Could you check a few things on this model? Use its own coordinates, in mm. Round coordinates to 2 decimals unless told otherwise and drop trailing zeros. Loops run counter-clockwise (first coordinate to the right, second up) from the corner with the lowest first, then second, coordinate; pieces in that order, holes last. Notation, with made-up numbers: (12.5, 26.25) -> (55.5, 26.25) arc R16 ccw to (55.5, 50.25) -> close; hole circle Ø6 at (15.5, 49). An arc over 180 degrees is marked (long way). Write each question's results on one line, items separated by ' | '.
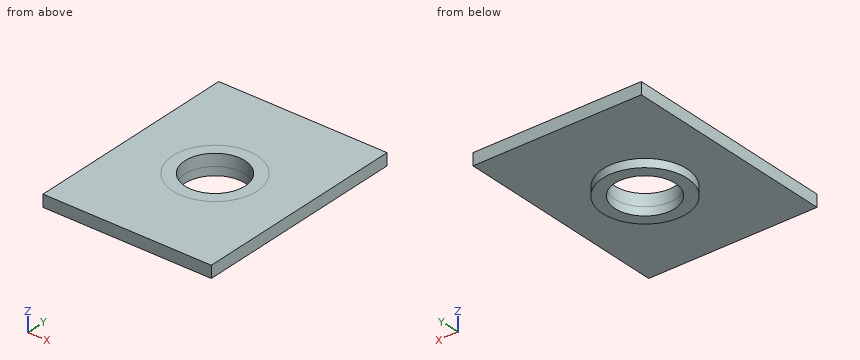
from build123d import *

# Parameters (mm, degrees)
CROQUIS1_R              = 35
SALIENTE_EXTRUIR1_DEPTH = 10
CROQUIS2_R              = 35
CROQUIS2_R_2            = 25
SALIENTE_EXTRUIR2_DEPTH = 7
SALIENTE_EXTRUIR4_START = -10
CROQUIS3_R              = 35
CROQUIS3_R_2            = 25
SALIENTE_EXTRUIR4_DEPTH = 10


with BuildPart() as part:
    # Croquis1 → Saliente-Extruir1 (new body)
    with BuildSketch(Plane.XY):
        Polygon((0, 0), (140, 0), (140, 180), (0, 180), (0, 49.177666069), align=None)
        with Locations((70, 90)):
            Circle(CROQUIS1_R, mode=Mode.SUBTRACT)
    extrude(amount=SALIENTE_EXTRUIR1_DEPTH)



with BuildPart() as body_2:
    # Croquis2 → Saliente-Extruir2 (new body)
    with BuildSketch(Plane(origin=(0, 0, 0), x_dir=(-1, 0, 0), z_dir=(0, 0, -1))):
        with Locations(Location((-70, 90, 0), (0, 0, 180))):
            Circle(CROQUIS2_R)
        with Locations((-70, 90)):
            Circle(CROQUIS2_R_2, mode=Mode.SUBTRACT)
    extrude(amount=SALIENTE_EXTRUIR2_DEPTH)


with BuildPart() as part_1:
    add(part.part)

    add(body_2.part)  # Saliente-Extruir4 merges body 2
    # Croquis3 → Saliente-Extruir4 (add)
    with BuildSketch(Plane.XY.offset(10).offset(SALIENTE_EXTRUIR4_START)):
        with Locations((70, 90)):
            Circle(CROQUIS3_R)
        with Locations((70, 90)):
            Circle(CROQUIS3_R_2, mode=Mode.SUBTRACT)
    extrude(amount=SALIENTE_EXTRUIR4_DEPTH)


solid = part_1.part
1) I want a section at C-C, the plane z = 2.75. Write out the boundary of the cut face in (x, y), plus the area to 3 significant figures.
Model answer:
outline: (0, 0) -> (140, 0) -> (140, 180) -> (0, 180) -> close; hole circle Ø50 at (70, 90) | area: 23,200 mm2
2) I'm going to push a flat-ended pin straight in: pin 1 (3 mm diameter, centred on x = 110.5, y = 91, fed in from -Z). Where does the tip first touch, or does it pass through?
Model answer:
pin 1: stops at z = 0
3) I want a section at D-D, the plane y = 62. Write out the boundary of the cut face in (x, z).
Model answer:
outline: (0, 0) -> (49, 0) -> (49, -7) -> (91, -7) -> (91, 0) -> (140, 0) -> (140, 10) -> (0, 10) -> close
4) I want a section at A-A, the plane y = 90. Write out the boundary of the cut face in (x, z).
Model answer:
outline: (0, 0) -> (35, 0) -> (35, -7) -> (45, -7) -> (45, 10) -> (0, 10) -> close; (95, -7) -> (105, -7) -> (105, 0) -> (140, 0) -> (140, 10) -> (95, 10) -> close
5) I need wall thicknesses on line 1 (X direction, y = 90, z = 7.75); line 2 (Y direction, x = 70, z = -2.25); line 3 (Z direction, x = 13.5, y = 149). Which ranges of each line are inside material? Lowest first, please.
Model answer:
line 1: x = 0 to 45, 95 to 140 | line 2: y = 55 to 65, 115 to 125 | line 3: z = 0 to 10
6) I want a section at B-B, the plane x = 70. Write out the boundary of the cut face in (y, z), plus the area to 3 significant figures.
Model answer:
outline: (0, 0) -> (55, 0) -> (55, -7) -> (65, -7) -> (65, 10) -> (0, 10) -> close; (115, -7) -> (125, -7) -> (125, 0) -> (180, 0) -> (180, 10) -> (115, 10) -> close | area: 1,440 mm2
